Autodesk Inventor part; units mm, degrees
ref_plane "YZ Plane" through (0, 0, 0) normal (1, 0, 0) x (0, 1, 0)
ref_plane "XZ Plane" through (0, 0, 0) normal (0, 1, 0) x (-1, 0, 0)
ref_plane "XY Plane" through (0, 0, 0) normal (0, 0, 1) x (1, 0, 0)
sketch "Sketch1" plane through (0, 0, 0) normal (0, 0, 1) x (1, 0, 0)
  line L0 (0, 0) -> (0, 25)
  line L1 (0, 25) -> (125, 25)
  line L2 (125, 25) -> (125, 0)
  line L3 (123, 0) -> (123, 23)
  line L4 (123, 23) -> (2, 23)
  line L5 (2, 23) -> (2, 0)
  line L6 (0, 0) -> (2, 0)
  line L7 (123, 0) -> (125, 0)
  dimension "d0" = 25
  dimension "d1" = 125
  dimension "d2" = 25
  dimension "d3" = 2
extrude "Extrusion1" add sketch "Sketch1" along normal mid plane 310
sketch "Sketch2" plane through (125, 0, 155) normal (1, 0, 0) x (0, 0, -1)
  line L0 (-37.205, -32.4182) -> (-16.8959, -51.5992)
  arc A0 (-19.2763, -56.7631) -> (-16.8959, -51.5992) centre (-18.9558, -53.7803) ccw
  line L1 (-19.2763, -56.7631) -> (-50.7848, -53.3777)
  arc A1 (-50.7848, -53.3777) -> (-55.7745, -43.3621) centre (-69.9997, -56.6998) ccw
  line L2 (-55.7745, -43.3621) -> (-48.1388, -31.7992)
  arc A2 (-48.1388, -31.7992) -> (-37.205, -32.4182) centre (-41.913, -18.7038) ccw
  line L3 (-75.1262, -21.5392) -> (-58.4114, -21.5392)
  arc A3 (-55.5831, -23.5388) -> (-58.4114, -21.5392) centre (-58.4114, -24.5392) ccw
  arc A4 (-55.5831, -23.5388) -> (-54.0148, -26.691) centre (-41.913, -18.7038) ccw
  arc A5 (-54.0941, -30.1103) -> (-54.0148, -26.691) centre (-56.5186, -28.3435) ccw
  line L4 (-54.0941, -30.1103) -> (-59.464, -37.4794)
  arc A6 (-62.97, -38.511) -> (-59.464, -37.4794) centre (-61.8885, -35.7127) ccw
  arc A7 (-62.97, -38.511) -> (-89.4714, -57.7495) centre (-69.9997, -56.6998) ccw
  arc A8 (-91.9686, -60.8693) -> (-89.4714, -57.7495) centre (-92.4671, -57.911) ccw
  arc A9 (-94.9644, -58.0288) -> (-91.9686, -60.8693) centre (-91.9686, -57.8693) ccw
  arc A10 (-90.8616, -42.9236) -> (-94.9644, -58.0288) centre (-69.9997, -56.6998) ccw
  line L5 (-90.8616, -42.9236) -> (-77.6297, -22.886)
  arc A11 (-75.1262, -21.5392) -> (-77.6297, -22.886) centre (-75.1262, -24.5392) ccw
  line L6 (14.2226, -42.1262) -> (14.481, -34.3473)
  arc A12 (16.1692, -31.7481) -> (14.481, -34.3473) centre (17.4793, -34.4469) ccw
  arc A13 (16.1692, -31.7481) -> (22.7187, -25.3606) centre (9.837, -18.7038) ccw
  arc A14 (25.3838, -23.7379) -> (22.7187, -25.3606) centre (25.3838, -26.7379) ccw
  line L7 (25.3838, -23.7379) -> (32.9823, -23.7379)
  arc A15 (35.8164, -27.7217) -> (32.9823, -23.7379) centre (32.9823, -26.7379) ccw
  arc A16 (20.9479, -43.8593) -> (35.8164, -27.7217) centre (9.837, -18.7038) ccw
  line L8 (20.9479, -43.8593) -> (18.4331, -44.97)
  arc A17 (14.2226, -42.1262) -> (18.4331, -44.97) centre (17.221, -42.2258) ccw
  arc A18 (-58.5566, -72.4892) -> (-51.863, -63.8628) centre (-69.9997, -56.6998) ccw
  arc A19 (-48.6463, -61.9952) -> (-51.863, -63.8628) centre (-49.0727, -64.9648) ccw
  line L9 (-48.6463, -61.9952) -> (-37.4684, -63.6003)
  arc A20 (-36.6827, -69.3141) -> (-37.4684, -63.6003) centre (-37.8948, -66.5698) ccw
  line L10 (-36.6827, -69.3141) -> (-55.5841, -77.6626)
  arc A21 (-58.5566, -72.4892) -> (-55.5841, -77.6626) centre (-56.7962, -74.9183) ccw
  arc A22 (-88.4942, -73.521) -> (-79.2774, -79.9145) centre (-69.9997, -56.6998) ccw
  arc A23 (-87.0146, -70.1753) -> (-88.4942, -73.521) centre (-87.0146, -72.1753) ccw
  arc A24 (-83.5364, -70.7358) -> (-84.9248, -70.1753) centre (-84.9248, -72.1753) ccw
  arc A25 (-83.5364, -70.7358) -> (-77.7157, -74.6082) centre (-69.9997, -56.6998) ccw
  arc A26 (-76.5074, -76.4798) -> (-77.7157, -74.6082) centre (-78.5071, -76.445) ccw
  line L11 (14.545, -2.9927) -> (14.545, 4.5521)
  arc A27 (18.4889, 7.3998) -> (14.545, 4.5521) centre (17.545, 4.5521) ccw
  arc A28 (35.8164, -9.6858) -> (18.4889, 7.3998) centre (9.837, -18.7038) ccw
  arc A29 (32.9823, -13.6696) -> (35.8164, -9.6858) centre (32.9823, -10.6696) ccw
  line L12 (32.9823, -13.6696) -> (25.3838, -13.6696)
  arc A30 (22.7187, -12.0469) -> (25.3838, -13.6696) centre (25.3838, -10.6696) ccw
  arc A31 (22.7187, -12.0469) -> (16.2237, -5.6861) centre (9.837, -18.7038) ccw
  arc A32 (14.545, -2.9927) -> (16.2237, -5.6861) centre (17.545, -2.9927) ccw
  line L13 (-41.913, 8.7962) -> (-41.4149, 8.7962)
  arc A33 (-38.601, 4.7561) -> (-41.4149, 8.7962) centre (-41.4149, 5.7962) ccw
  line L14 (-38.601, 4.7561) -> (-41.237, -2.375)
  arc A34 (-43.6844, -4.3124) -> (-41.237, -2.375) centre (-44.0509, -1.3349) ccw
  arc A35 (-43.6844, -4.3124) -> (-55.5831, -13.8687) centre (-41.913, -18.7038) ccw
  arc A36 (-58.4114, -15.8684) -> (-55.5831, -13.8687) centre (-58.4114, -12.8684) ccw
  line L15 (-58.4114, -15.8684) -> (-67.4194, -15.8684)
  arc A37 (-69.9228, -11.2152) -> (-67.4194, -15.8684) centre (-67.4194, -12.8684) ccw
  line L16 (-69.9228, -11.2152) -> (-64.861, -3.5499)
  arc A38 (-41.913, 8.7962) -> (-64.861, -3.5499) centre (-41.913, -18.7038) ccw
  line L17 (-27.9232, -22.5166) -> (-4.1527, -22.5166)
  arc A39 (-4.1527, -22.5166) -> (3.5036, -31.7475) centre (9.837, -18.7038) ccw
  arc A40 (5.1099, -35.1484) -> (3.5036, -31.7475) centre (2.1933, -34.4462) ccw
  line L18 (5.1099, -35.1484) -> (1.9297, -48.3572)
  arc A41 (-2.7527, -50.0803) -> (1.9297, -48.3572) centre (-0.9869, -47.6549) ccw
  line L19 (-2.7527, -50.0803) -> (-31.7052, -29.0019)
  arc A42 (-31.7052, -29.0019) -> (-27.9232, -22.5166) centre (-41.913, -18.7038) ccw
  line L20 (-6.2824, -14.891) -> (-25.7935, -14.891)
  arc A43 (-28.5569, -13.0589) -> (-25.7935, -14.891) centre (-25.7935, -11.891) ccw
  arc A44 (-28.5569, -13.0589) -> (-34.5765, -6.1967) centre (-41.913, -18.7038) ccw
  arc A45 (-35.7016, -2.1898) -> (-34.5765, -6.1967) centre (-33.0586, -3.6091) ccw
  line L21 (-35.7016, -2.1898) -> (-30.651, 7.2155)
  arc A46 (-28.008, 8.7962) -> (-30.651, 7.2155) centre (-28.008, 5.7962) ccw
  line L22 (-28.008, 8.7962) -> (-0.2731, 8.7962)
  arc A47 (2.7269, 5.7962) -> (-0.2731, 8.7962) centre (-0.2731, 5.7962) ccw
  line L23 (2.7269, 5.7962) -> (2.7269, -4.4197)
  arc A48 (1.46, -6.8684) -> (2.7269, -4.4197) centre (-0.2731, -4.4197) ccw
  arc A49 (1.46, -6.8684) -> (-3.5191, -13.0589) centre (9.837, -18.7038) ccw
  arc A50 (-6.2824, -14.891) -> (-3.5191, -13.0589) centre (-6.2824, -11.891) ccw
  circle A51 centre (-81.913, -5.781) radius 2.75
  circle A52 centre (7.837, -58.4172) radius 2.75
  circle A53 centre (-19.913, 17.776) radius 2.75
  circle A54 centre (-109.9997, -47.6996) radius 2.75
  circle A55 centre (43.4223, 4.8129) radius 2.75
  line L24 (-25.906, 18.0659) -> (-40.1014, 18.7524)
  arc A56 (-40.1014, 18.7524) -> (-73.2057, 1.9606) centre (-41.913, -18.7038) ccw
  line L25 (-73.2057, 1.9606) -> (-74.4501, 0.0761)
  arc A57 (-78.6067, -0.7742) -> (-82.3668, 0.2018) centre (-81.913, -5.781) ccw
  line L26 (-85.6456, -16.8777) -> (-99.2063, -37.4131)
  arc A58 (-99.2063, -37.4131) -> (-100.1023, -38.8439) centre (-69.9997, -56.6998) ccw
  arc A59 (-113.4192, -52.6298) -> (-109.9997, -53.6996) centre (-109.9997, -47.6996) ccw
  line L27 (-109.9997, -53.6996) -> (-107.9997, -53.6996)
  arc A60 (-104.9997, -56.6996) -> (-54.959, -88.3032) centre (-69.9997, -56.6998) ccw
  line L28 (-54.959, -88.3032) -> (2.4193, -60.9957)
  arc A61 (2.4193, -60.9957) -> (13.2548, -55.8388) centre (7.837, -58.4172) ccw
  line L29 (13.2548, -55.8388) -> (24.8778, -50.3072)
  arc A62 (24.8778, -50.3072) -> (42.845, -7.0644) centre (9.837, -18.7038) ccw
  line L30 (42.845, -7.0644) -> (48.4494, 1.5375)
  arc A63 (48.4494, 1.5375) -> (42.0639, 10.6571) centre (43.4223, 4.8129) ccw
  line L31 (42.0639, 10.6571) -> (32.0639, 8.3327)
  arc A64 (32.0639, 8.3327) -> (11.5279, 16.2554) centre (9.837, -18.7038) ccw
  line L32 (11.5279, 16.2554) -> (-13.92, 17.4862)
  arc A65 (-13.92, 17.4862) -> (-25.906, 18.0659) centre (-19.913, 17.776) ccw
  circle A66 centre (-69.9997, -56.6998) radius 9.5
  circle A67 centre (-41.913, -18.7038) radius 9.5
  circle A68 centre (9.837, -18.7038) radius 9.5
  circle A69 centre (35, 17) radius 2.75
  circle A70 centre (155, 12.5) radius 2.75
  line L33 (155, 0) -> (155, 25)
  line L34 (0, 25) -> (310, 25)
  line L35 (0, 0) -> (0, 25)
  circle A71 centre (266.5777, 4.8129) radius 2.75
  circle A72 centre (275, 17) radius 2.75
  circle A73 centre (155, 12.5) radius 2.75
  circle A74 centre (-106.7656, -26.4398) radius 1.65
  arc A75 (-104.9997, -56.6996) -> (-107.9997, -53.6996) centre (-107.9997, -56.6996) ccw
  arc A76 (-78.6067, -0.7742) -> (-74.4501, 0.0761) centre (-76.9535, 1.7293) ccw
  line L36 (-82.3668, 0.2018) -> (-122.8325, -2.8676)
  arc A77 (-122.8325, -2.8676) -> (-132.7182, -39.2443) centre (-121.3198, -22.8103) ccw
  line L37 (-132.7182, -39.2443) -> (-113.4192, -52.6298)
  circle A78 centre (-131.7402, -33.5999) radius 1.65
  circle A79 centre (-121.3198, -22.8103) radius 10.5
  circle A80 centre (-125.4537, -8.3911) radius 1.65
  line L38 (-104.3923, -39.7785) -> (-104.8988, -39.4272)
  arc A81 (-105.5539, -35.1162) -> (-104.8988, -39.4272) centre (-103.189, -36.9621) ccw
  arc A82 (-105.5539, -35.1162) -> (-102.1972, -16.9514) centre (-121.3198, -22.8103) ccw
  arc A83 (-99.5557, -13.0811) -> (-102.1972, -16.9514) centre (-99.3288, -16.0725) ccw
  line L39 (-99.5557, -13.0811) -> (-88.3759, -12.2331)
  arc A84 (-85.6456, -16.8777) -> (-88.3759, -12.2331) centre (-88.149, -15.2245) ccw
  arc A85 (-104.3923, -39.7785) -> (-100.1023, -38.8439) centre (-102.6826, -37.3134) ccw
  line L40 (-76.5074, -76.4798) -> (-76.5355, -78.0922)
  arc A86 (-79.2774, -79.9145) -> (-76.5355, -78.0922) centre (-78.5352, -78.0573) ccw
  line L41 (-87.0146, -70.1753) -> (-84.9248, -70.1753)
  point P0 (-69.9997, -56.6998)
  point P1 (-69.9997, -56.6998)
  point P2 (-69.9997, -56.6998)
  point P3 (-69.9997, -56.6998)
  point P4 (-107.9997, -56.6996)
  point P5 (-102.6826, -37.3134)
  point P6 (-69.9997, -56.6998)
  dimension "d6" = 5.5
  dimension "d7" = 5.5
  dimension "d8" = 8
  dimension "d9" = 12.5
  dimension "d10" = 35
extrude "Extrusion2" cut sketch "Sketch2" against normal blind 205.75 contours A70 L33 | L33 A70 | A55 | A69 | A71 | A72
sketch "Sketch3" plane through (0, 25, 155) normal (0, 1, 0) x (1, 0, 0)
  circle A0 centre (62.5, 60) radius 40
  line L0 (125, 0) -> (125, 310)
  line L1 (125, 0) -> (0, 0)
  circle A1 centre (62.5, 250) radius 40
  line L2 (0, 310) -> (125, 310)
  circle A2 centre (62.5, 155) radius 40
  point P0 (0, 155)
  dimension "d13" = 80
  dimension "d14" = 62.5
  dimension "d15" = 60
  dimension "d16" = 80
  dimension "d17" = 62.5
  dimension "d18" = 60
  dimension "d19" = 80
  dimension "d20" = 62.5
  dimension "d21" = 155
extrude "Extrusion3" cut sketch "Sketch3" against normal blind 10
properties part number "Mottor Protection Piece" material "Aluminum 6061"
CAD build for the part. Positions are in the model's coordinates, mm. A direction names the side the tool comes from. Give positions to 0.01 mm unless a question says otherwise; leave off trailing zeros. Order: outer loops, then holes, each group sorted by start corner. A loop starts at its lowest first (then second) coordinate and runs counter-clockwise, first axis right, second up. Notation, with made-up numbers: (52.25, 84) -> (111.25, 84) arc R24 ccw to (111.25, 111) -> close; hole circle Ø1 at (-40, 1). An arc over 180 degrees is marked (long way). Return JSON: item names as keys, results as strings.
Q1. Saw through at D-D (x = 70). Write the cut outline in (y, z), then the cut area to 3 significant figures.
Working result:
{"outline": "(23, -155) -> (25, -155) -> (25, -134.29) -> (23, -134.29) -> close; (23, -55.71) -> (25, -55.71) -> (25, -39.29) -> (23, -39.29) -> close; (23, 39.29) -> (25, 39.29) -> (25, 55.71) -> (23, 55.71) -> close; (23, 134.29) -> (25, 134.29) -> (25, 155) -> (23, 155) -> close", "area": "149 mm²"}
Q2. Which spindle directions (+Z, -Z, +X, -X, +Y, -Y) get a long thin tool onto all of the face, cutting with end or side? Do faces 4 (the face through (125, 10, -2)), 5 (the face through (2, 9, -2)). Say none if no direction does.
Working result:
{"face 4": "+Z, -Z, +X, +Y, -Y", "face 5": "+Z, -Z, -Y"}
Q3. Mould opens along Z. For faces 1 (the face through (62, 24, -155)), 2 (the face through (124.014, 14.359, 2.027)), 3 (the face through (0, 10, -2)) say: pulls with the +Z half, pulls with the -Z half, needs draft (parallel to the pull), parting line crosses it, or undercut.
Working result:
{"face 1": "pulls with the -Z half", "face 2": "undercut", "face 3": "needs draft"}
Q4. Saw through at C-C (z = 95). Write the cut outline in (x, y), then the cut area to 3 significant figures.
Working result:
{"outline": "(0, 0) -> (2, 0) -> (2, 23) -> (22.5, 23) -> (22.5, 25) -> (0, 25) -> close; (102.5, 23) -> (123, 23) -> (123, 0) -> (125, 0) -> (125, 25) -> (102.5, 25) -> close", "area": "182 mm²"}
Q5. Saw through at B-B (x = 32). Write the cut outline in (y, z), then the cut area to 3 significant figures.
Working result:
{"outline": "(23, -155) -> (25, -155) -> (25, -120.88) -> (23, -120.88) -> close; (23, -69.12) -> (25, -69.12) -> (25, -25.88) -> (23, -25.88) -> close; (23, 25.88) -> (25, 25.88) -> (25, 69.12) -> (23, 69.12) -> close; (23, 120.88) -> (25, 120.88) -> (25, 155) -> (23, 155) -> close", "area": "309 mm²"}
Q6. Drill centre lines: line 1 (X direction, y = 1.75, z = 139.5); line 2 (Z direction, x = 62.5, y = 24.15); line 3 (Y direction, x = 1, z = 120). Where is each one in solid material? Low to high.
Working result:
{"line 1": "0 to 2, 123 to 125", "line 2": "-155 to -135, -55 to -40, 40 to 55, 135 to 155", "line 3": "0 to 14.25, 19.75 to 25"}
Q7. Flat gauge pins, fed straight in: pin 1 (6.5 mm diameter, centred on y = 4.81, z = 111.58, fed in from +X); pin 2 (3.5 mm diameter, centred on y = 17, z = -120, fed in from -X); pin 3 (5 mm diameter, centred on x = 25, z = 50.5, fed in from -Y). Where does each tip first touch, or does it go through?
Working result:
{"pin 1": "x = 125", "pin 2": "through", "pin 3": "y = 23"}
Q8. Saw through at A-A (z = 0). Write the cut outline in (x, y).
Working result:
{"outline": "(0, 0) -> (2, 0) -> (2, 9.75) -> (0, 9.75) -> close; (0, 15.25) -> (2, 15.25) -> (2, 23) -> (22.5, 23) -> (22.5, 25) -> (0, 25) -> close; (102.5, 23) -> (123, 23) -> (123, 15.25) -> (125, 15.25) -> (125, 25) -> (102.5, 25) -> close; (123, 0) -> (125, 0) -> (125, 9.75) -> (123, 9.75) -> close"}
